Source: CAD feature listing. Evaluate the final solid. Frame: model axes, mm. A direction names the side the tool comes from. Give positions to 0.01 mm unless a question says otherwise; leave off trailing zeros. Order: outer loops, then holes, each group sorted by start corner. A loop starts at its lowest first (then second) coordinate and runs counter-clockwise, first axis right, second up.
```python
from build123d import *

# Parameters (mm, degrees)
SKETCH_1_R            = 37.25
SKETCH_1_R_2          = 33.5
MAIN_DEPTH            = 25
SKETCH_3_R            = 33.5
SKETCH_3_R_2          = 5
STOP_DEPTH            = 5
LOCK_DEPTH            = 25
SKETCH_5_W            = 6
SKETCH_5_H            = 48.380798507
SLOT_DEPTH            = 25
SKETCH_6_R            = 2.25
SMALL_HOLES_DEPTH     = 71.804407802
HOLES_FOR_BOLTS_REACH = 66.252
SKETCH_7_R            = 2
HEXAGONS_DEPTH        = 2


with BuildPart() as part:
    # Эскиз1 → main (new body)
    with BuildSketch(Plane(origin=(0, 0, 0), x_dir=(1, 0, 0), z_dir=(0, 1, 0))):
        with Locations(Location((0, 0, 0), (0, 0, 90))):
            Circle(SKETCH_1_R)
        with Locations(Location((0, 0, 0), (0, 0, 270))):
            Circle(SKETCH_1_R_2, mode=Mode.SUBTRACT)
    extrude(amount=MAIN_DEPTH)

    # Эскиз3 → stop (add)
    with BuildSketch(Plane(origin=(0, 0, 0), x_dir=(1, 0, 0), z_dir=(0, 1, 0))):
        with Locations(Location((0, 0, 0), (0, 0, 270))):
            Circle(SKETCH_3_R)
        with Locations(Location((0, 0, 0), (0, 0, 270))):
            Circle(SKETCH_3_R_2, mode=Mode.SUBTRACT)
    extrude(amount=STOP_DEPTH)

    # Эскиз4 → lock (add)
    with BuildSketch(Plane(origin=(0, 0, 0), x_dir=(1, 0, 0), z_dir=(0, 1, 0))):
        with BuildLine():
            Line((-8, -36.380798507), (-8, -48.380798507))
            Line((-8, -48.380798507), (8, -48.380798507))
            Line((8, -48.380798507), (8, -36.380798507))
            ThreePointArc((8, -36.380798507), (0, -37.25), (-8, -36.380798507))
        make_face()
    extrude(amount=LOCK_DEPTH)

    # Эскиз5 → slot (cut)
    with BuildSketch(Plane(origin=(0, 0, 0), x_dir=(1, 0, 0), z_dir=(0, 1, 0))):
        with Locations((0, -24.190399254)):
            Rectangle(SKETCH_5_W, SKETCH_5_H)
    extrude(amount=SLOT_DEPTH, mode=Mode.SUBTRACT)

    # Эскиз6 → small holes (cut, through all)
    with BuildSketch(Plane(origin=(8, 0, 0), x_dir=(0, 0, -1), z_dir=(1, 0, 0))):
        with Locations((-42.380798507, 7)):
            Circle(SKETCH_6_R)
        with Locations((-42.380798507, 18)):
            Circle(SKETCH_6_R)
    extrude(amount=-SMALL_HOLES_DEPTH, mode=Mode.SUBTRACT)

    # Эскиз7 → holes for bolts (cut, up to next)
    with BuildSketch(Plane(origin=(0, 5, 0), x_dir=(1, 0, 0), z_dir=(0, 1, 0)), mode=Mode.PRIVATE) as holes_for_bolts_sk1:
        with Locations(Location((0, 12.5, 0), (0, 0, 270))):
            Circle(SKETCH_7_R)
    holes_for_bolts_tool1 = extrude(holes_for_bolts_sk1.sketch, amount=-HOLES_FOR_BOLTS_REACH, mode=Mode.PRIVATE) & part.part
    # Эскиз7 → holes for bolts (cut, up to next)
    with BuildSketch(Plane(origin=(0, 5, 0), x_dir=(1, 0, 0), z_dir=(0, 1, 0)), mode=Mode.PRIVATE) as holes_for_bolts_sk2:
        with Locations(Location((-10.825317547, -6.25, 0), (0, 0, 270))):
            Circle(SKETCH_7_R)
    holes_for_bolts_tool2 = extrude(holes_for_bolts_sk2.sketch, amount=-HOLES_FOR_BOLTS_REACH, mode=Mode.PRIVATE) & part.part
    # Эскиз7 → holes for bolts (cut, up to next)
    with BuildSketch(Plane(origin=(0, 5, 0), x_dir=(1, 0, 0), z_dir=(0, 1, 0)), mode=Mode.PRIVATE) as holes_for_bolts_sk3:
        with Locations(Location((10.825317547, -6.25, 0), (0, 0, 90))):
            Circle(SKETCH_7_R)
    holes_for_bolts_tool3 = extrude(holes_for_bolts_sk3.sketch, amount=-HOLES_FOR_BOLTS_REACH, mode=Mode.PRIVATE) & part.part
    add(holes_for_bolts_tool1.solids().sort_by_distance((0, 5, -12.5))[0], mode=Mode.SUBTRACT)
    add(holes_for_bolts_tool2.solids().sort_by_distance((-10.825318, 5, 6.25))[0], mode=Mode.SUBTRACT)
    add(holes_for_bolts_tool3.solids().sort_by_distance((10.825318, 5, 6.25))[0], mode=Mode.SUBTRACT)

    # Эскиз8 → hexagons (cut)
    with BuildSketch(Plane(origin=(0, 5, 0), x_dir=(1, 0, 0), z_dir=(0, 1, 0))):
        Polygon((-8.575317547, -10.147114317), (-6.325317547, -6.25), (-8.575317547, -2.352885683), (-13.075317547, -2.352885683), (-15.325317547, -6.25), (-13.075317547, -10.147114317), align=None)
        Polygon((13.075317547, -10.147114317), (15.325317547, -6.25), (13.075317547, -2.352885683), (8.575317547, -2.352885683), (6.325317547, -6.25), (8.575317547, -10.147114317), align=None)
        Polygon((2.25, 8.602885683), (4.5, 12.5), (2.25, 16.397114317), (-2.25, 16.397114317), (-4.5, 12.5), (-2.25, 8.602885683), align=None)
    extrude(amount=-HEXAGONS_DEPTH, mode=Mode.SUBTRACT)


solid = part.part
```
1) Section query B-B, the plane y = 18. Return the cut outline in (x, z), and give its area (3 significant figures).
Report:
outline: (-8, 36.38) arc R37.25 ccw (long way) to (8, 36.38) - (8, 40.13) - (3, 40.13) - (3, 33.37) arc R33.5 cw (long way) to (-3, 33.37) - (-3, 40.13) - (-8, 40.13) - close; (-8, 44.63) - (-3, 44.63) - (-3, 48.38) - (-8, 48.38) - close; (3, 44.63) - (8, 44.63) - (8, 48.38) - (3, 48.38) - close
area: 882 mm2
2) Material intervals for L1, parallel to X at y = 3.35, z = 0; L2, parallel to X at y = 6.75, z = 1; L3, parallel to Y at x = 23, z = -22, sorted ascending.
Report:
L1: x = -37.25 to -5, 5 to 37.25
L2: x = -37.24 to -33.49, 33.49 to 37.24
L3: y = 0 to 5
3) Section query A-A, the plane x = 0. Return the cut outline in (y, z), and give its area (3 significant figures).
Report:
outline: (0, -37.25) - (25, -37.25) - (25, -33.5) - (5, -33.5) - (5, -16.4) - (3, -16.4) - (3, -14.5) - (0, -14.5) - close; (0, -10.5) - (3, -10.5) - (3, -8.6) - (5, -8.6) - (5, -5) - (0, -5) - close
area: 209 mm2
4) Draft query along Y for faces 1 (the flat face through (-3, 10, 36)), 2 (the cylindrical face through (5.535, 16.004, 41.343)), 3 (the flat face through (-7, 5, -1)). Return one class per face: +Y half, -Y half, draft (parallel to the pull), parting line (faces both ways), or undercut.
Report:
face 1: draft
face 2: undercut
face 3: +Y half
5) Reachability of faces 4 (the flat face through (8, 12, 42)), 5 (the flat face through (-7.435, 4.014, 4.329)), 6 (the cylindrical face through (9.47, 1.52, 7.72)) from +Z, -Z, +X, -X, +Y, -Y: full face, straight path, thin tool, end or side. Return the list, or none.
Report:
face 4: +Z, +X, +Y, -Y
face 5: +Y
face 6: +Y, -Y
6) Section query D-D, the plane z = 42.5. Return the cut outline in (x, y), and give its area (3 significant figures).
Report:
outline: (-8, 0) - (-3, 0) - (-3, 4.75) - (-8, 4.75) - close; (-8, 9.25) - (-3, 9.25) - (-3, 15.75) - (-8, 15.75) - close; (-8, 20.25) - (-3, 20.25) - (-3, 25) - (-8, 25) - close; (3, 0) - (8, 0) - (8, 4.75) - (3, 4.75) - close; (3, 9.25) - (8, 9.25) - (8, 15.75) - (3, 15.75) - close; (3, 20.25) - (8, 20.25) - (8, 25) - (3, 25) - close
area: 160 mm2
7) Pin query (flat end, axial travel): pin 1 (2 mm diameter, centred on x = 1.5, y = 16.5, fed in from -Z); pin 2 (3.5 mm diameter, centred on y = 15.5, z = 41.5, fed in from +X); pin 3 (5 mm diameter, centred on y = 11, z = 28.5, fed in from +X). Return the tip coordinate at first contact, or that it passes through.
Report:
pin 1: stops at z = -37.25
pin 2: stops at x = 8
pin 3: stops at x = 26.68
8) Section query C-C, the plane z = 0. Return the cut outline in (x, y).
Report:
outline: (-37.25, 0) - (-5, 0) - (-5, 5) - (-33.5, 5) - (-33.5, 25) - (-37.25, 25) - close; (5, 0) - (37.25, 0) - (37.25, 25) - (33.5, 25) - (33.5, 5) - (5, 5) - close
